```python
from build123d import *

# Parameters (mm, degrees)
F1_DEPTH = 25.4
F2_R     = 20.781866
F3_DEPTH = 17.769353
F4_DEPTH = 11.559019
F5_DEPTH = 25.4
F6_T     = -2.54
F7_DEPTH = 8.098027


with BuildPart() as f1:
    # F0 (on Front) → F1 (new body)
    with BuildSketch(Plane.XZ):
        Polygon((35.715379, 0), (19.829497, 35.855889), (-21.848936, 35.855889), (-37.045002, 0), (0, 0), align=None)
    extrude(amount=F1_DEPTH)

    # F2 (on Top) → F3 (join)
    with BuildSketch(Plane.XY):
        Circle(F2_R)
    extrude(amount=-F3_DEPTH)

    # F3_face (on face) → F4 (join)
    with BuildSketch(Plane(origin=(0, 8.820098, 0), x_dir=(1, 0, 0), z_dir=(0, 0, 1))):
        with BuildLine():
            Line((-20.781866, -8.820098), (20.781866, -8.820098))
            ThreePointArc((20.781866, -8.820098), (0, 11.961768), (-20.781866, -8.820098))
        make_face()
    extrude(amount=F4_DEPTH)

    # F0 (on Front) → F5 (join)
    with BuildSketch(Plane.XZ):
        Polygon((35.715379, 0), (19.829497, 35.855889), (-21.848936, 35.855889), (-37.045002, 0), (0, 0), align=None)
    extrude(amount=-F5_DEPTH)

    # F6
    f6_openings = [f1.faces().sort_by_distance(p)[0] for p in [
        (-0.821653, -25.4, 16.304849),
        (-0.821653, 25.4, 16.304849),
    ]]
    offset(amount=F6_T, openings=f6_openings)

    # F2 (on Top) → F7 (join)
    with BuildSketch(Plane.XY):
        Circle(F2_R)
    extrude(amount=F7_DEPTH)


solid = f1.part
```
Verification items for the finished model (mm, model axes). A direction names the side the tool comes from. Round coordinates to 2 decimals unless told otherwise and drop trailing zeros. Write each loop counter-clockwise with the first axis right and the second up, starting at its lowest first coordinate (ties: lowest second). Pieces come first, ordered by that corner, then holes. Notation, with made-up numbers: (-32.75, 56.25) - (18.25, 56.25) arc R22 cw to (18.25, 83.25) - close; hole circle Ø11 at (35, 37). An arc over 180 degrees is marked (long way). Answer as a JSON object with one key per item and string values. Group by question number.
Q1. Section check B-B, the plane y = 0. Enter the section's corners in (x, z) (1 decimal).
Q2. Section check D-D, the plane x = -28.5. Enter the section's corners in (y, z).
Q3. Section check A-A, the plane x = 0. Enter the section's corners in (y, z).
Q4. Section check C-C, the plane z = 23.5. Enter the section's corners in (x, y), plus the area to 3 significant figures.
Q5. Mould release check, pull along Z, two halves, no side actions. Record for faces 5 (the cylindrical face through (-4.505, -20.288, -9.009)), 6 (the flat face through (-26.6, -0.36, 18.14)), 7 (the flat face through (27.884, -0.356, 17.677)): released by +Z, released by -Z, zero draft, split by the parting line, or undercut.
Q6. Tool access check on faces 1 (the flat face through (25.09, -0.36, 17.71)), 2 (the flat face through (0, 0, -17.769)), 3 (the flat face through (-1, -23, 0)), 4 (the flat face through (0, 0, 0)). Record the directions out of +Z, -Z, +X, -X, +Y, -Y that give a thin tool (end or side, any length) a straight path to the whole face; none if there is none.
Q7. Thickness scan on line 1 (Z direction, x = -19.5, y = 22.5); line 2 (Y direction, x = 0, z = -6); line 3 (Z direction, x = 3, y = -16.5). Record the ranges inside material, lowest first.
Q8. Go/stop test with flat-tipped pins: pin 1 Ø3 at (y, z) = (18, 9.5) entering from -X; pin 2 Ø12 at (x, y) = (-28.5, -1) entering from -Z; pin 3 Ø12 at (x, z) = (-8.5, -10) entering from +Y. Record where each tip stops, or that it passes through.
Found:
{
 "1": {"outline": "(-37, 0) - (-20.8, 0) - (-20.8, -17.8) - (20.8, -17.8) - (20.8, 0) - (35.7, 0) - (19.8, 35.9) - (-21.8, 35.9) - close; hole (-33.2, 2.5) - (-20.8, 2.5) - (-20.8, 8.1) - (20.8, 8.1) - (20.8, 2.5) - (31.8, 2.5) - (18.2, 33.3) - (-20.2, 33.3) - close; hole (-18.2, -15.2) - (18.2, -15.2) - (18.2, 0) - (-18.2, 0) - close"},
 "2": {"outline": "(-25.4, 0) - (25.4, 0) - (25.4, 2.54) - (-25.4, 2.54) - close; (-25.4, 13.65) - (25.4, 13.65) - (25.4, 20.16) - (-25.4, 20.16) - close"},
 "3": {"outline": "(-25.4, 0) - (-20.78, 0) - (-20.78, -17.77) - (20.78, -17.77) - (20.78, 0) - (25.4, 0) - (25.4, 2.54) - (20.78, 2.54) - (20.78, 8.1) - (-20.78, 8.1) - (-20.78, 2.54) - (-25.4, 2.54) - close; (-25.4, 33.32) - (25.4, 33.32) - (25.4, 35.86) - (-25.4, 35.86) - close; hole (-18.24, -15.23) - (18.24, -15.23) - (18.24, 0) - (-18.24, 0) - close"},
 "4": {"outline": "(-27.09, -25.4) - (-24.33, -25.4) - (-24.33, 25.4) - (-27.09, 25.4) - close; (22.53, -25.4) - (25.3, -25.4) - (25.3, 25.4) - (22.53, 25.4) - close", "area": "281 mm^2"},
 "5": {"face 5": "zero draft", "face 6": "undercut", "face 7": "released by +Z"},
 "6": {"face 1": "+Y, -Y", "face 2": "-Z, +X, -X, +Y, -Y", "face 3": "-Z", "face 4": "none"},
 "7": {"line 1": "z = 0 to 2.54, 33.32 to 35.86", "line 2": "y = -20.78 to -18.24, 18.24 to 20.78", "line 3": "z = -17.77 to -15.23, 0 to 8.1, 33.32 to 35.86"},
 "8": {"pin 1": "stops at x = -33.65", "pin 2": "stops at z = 0", "pin 3": "stops at y = 20.63"}
}
